Source: CAD feature listing. Evaluate the final solid. Frame: model axes, mm. Coordinates: 2 decimals unless noted, no trailing zeros. Loops run counter-clockwise (first coordinate to the right, second up) from the corner with the lowest first, then second, coordinate; pieces in that order, holes last. Notation, with made-up numbers: (-7, -16) -> (17, -16) arc R30 ccw to (17, 21) -> close; hole circle Ø3 at (27, 8). An arc over 180 degrees is marked (long way). Answer as CSV lines item,"result".
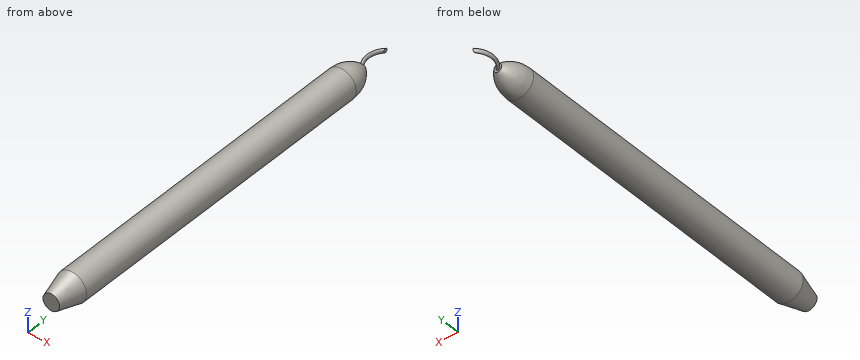
from build123d import *

# Parameters (mm, degrees)
SKETCH7_R = 2


with BuildPart() as part:
    # Sketch1 → Revolve1 (revolve)
    with BuildSketch(Plane.XY, mode=Mode.PRIVATE) as revolve1_sk:
        with BuildLine():
            Line((0, 0), (0, 380))
            Line((0, 380), (4, 380))
            ThreePointArc((4, 380), (12.132538026, 368.39895852), (15, 354.524521594))
            Line((15, 354.524521594), (15, 25))
            Line((15, 25), (8.301270189, 0))
            Line((8.301270189, 0), (0, 0))
        make_face()
    revolve(revolve1_sk.sketch.rotate(Axis((0, 0, 0), (0, 1, 0)), 90), axis=Axis((0, 0, 0), (0, 1, 0)))

    # Sweep6: sweep along a path in Sketch11
    with BuildLine(Plane.XY) as sweep6_path:
        ThreePointArc((0, 380), (-5.857864376, 394.142135624), (0, 408.284271247))
    # Sketch7 → Sweep6 (sweep)
    with BuildSketch(Plane(origin=(0, 380, 0), x_dir=(1, 0, 0), z_dir=(0, 1, 0))):
        Circle(SKETCH7_R)
    sweep(path=sweep6_path.line)


solid = part.part
(1) Cut plane A-A (y = 241). Return the cut outline in (x, z).
Computed values:
outline,"circle Ø30 at (0, 0)"
(2) Pin query (flat end, axial travel): pin 1 Ø1.5 at (x, z) = (11.5, 12) entering from +Y; pin 2 Ø5 at (x, z) = (-4, 0.5) entering from +Y; pin 3 Ø3 at (y, z) = (408.5, 0) entering from +X; pin 4 Ø8 at (x, z) = (10, -9) entering from +Y. Return the tip coordinate at first contact, or that it passes through.
Computed values:
pin 1,"through"
pin 2,"y = 408.81"
pin 3,"x = 0"
pin 4,"y = 373.43"
(3) Material intervals for L1, parallel to X at y = 33.5, z = 0; L2, parallel to Z at x = 7, y = 339; L3, parallel to Z at x = 1, y = 355.5, sorted ascending. Write a range as [from, to].
Computed values:
L1,"[-15, 15]"
L2,"[-13.27, 13.27]"
L3,"[-14.95, 14.95]"
